```python
from build123d import *

# Parameters (mm, degrees)
F0_W        = 23
F0_H        = 25
F1_DEPTH    = 1.2
F3_DEPTH    = 25
F5_W        = 1.3906080276
F5_H        = 1.7
F5_W_2      = 1.5159434646
F6_DEPTH    = 25
F7_T1_DEPTH = 30


# Not quite as in the source:
# - a fillet or chamfer that OpenCascade refuses, or shapes differently, is made with other operations: its cross-section is extruded or revolved along the edge and cut away or added


with BuildPart() as f1:
    # F0 (on Top) → F1 (new body)
    with BuildSketch(Plane.XY):
        Rectangle(F0_W, F0_H)
    extrude(amount=F1_DEPTH)

    # F2 (on face) → F3 (join)
    with BuildSketch(Plane.XZ.offset(12.5)):
        with BuildLine():
            ThreePointArc((-8.8198933508, 1.2), (-16.4322899898, -1.1691927474), (-13.6809007153, -8.6519404997))
            Line((-13.6809007153, -8.6519404997), (-13.1818733439, -6.6722285874))
            ThreePointArc((-13.1818733439, -6.6722285874), (-14.8938387487, -2.747327312), (-11.5259407878, -0.1029107612))
            Line((-11.5259407878, -0.1029107612), (-11.5, 0))
            Line((-11.5, 0), (-11.5, 1.2))
            Line((-11.5, 1.2), (-8.8198933508, 1.2))
        make_face()
        with BuildLine():
            ThreePointArc((17, -3.4602172673), (14.1631160155, 1.3520392811), (8.578977059, 1.2))
            Line((8.578977059, 1.2), (11.5, 1.2))
            Line((11.5, 1.2), (11.5, 0.0397827327))
            ThreePointArc((11.5, 0.0397827327), (13.9748737342, -0.9853435331), (15, -3.4602172673))
            ThreePointArc((15, -3.4602172673), (14.5929628971, -5.0983810311), (13.4665254188, -6.3555199764))
            Line((13.4665254188, -6.3555199764), (14.0745145934, -8.3204512748))
            ThreePointArc((14.0745145934, -8.3204512748), (16.2122091562, -6.2966031487), (17, -3.4602172673))
        make_face()
    extrude(amount=-F3_DEPTH)

    # F5 (on face) → F6 (join)
    with BuildSketch(Plane.XZ.offset(12.5)):
        with Locations((18.6200318858, 6.0247716144)):
            Rectangle(F5_W, F5_H)
        with BuildLine():
            ThreePointArc((16.5864266455, -1.367787106), (17, -3.4602172673), (16.5864266455, -5.5526474285))
            Line((16.5864266455, -5.5526474285), (16.5864266455, -6.6252283856))
            Line((16.5864266455, -6.6252283856), (17.924727872, -6.6252283856))
            Line((17.924727872, -6.6252283856), (17.924727872, 5.1747716144))
            Line((17.924727872, 5.1747716144), (17.924727872, 6.8747716144))
            Line((17.924727872, 6.8747716144), (16.5864266455, 6.8747716144))
            Line((16.5864266455, 6.8747716144), (16.5864266455, 1.253477479))
            Line((16.5864266455, 1.253477479), (16.5864266455, -1.367787106))
        make_face()
        Polygon((32.124727872, -6.6252283856), (33.5864266455, -6.6252283856), (33.5864266455, 6.8747716144), (32.124727872, 6.8747716144), (32.124727872, 5.1747716144), align=None)
        with Locations((31.3667561397, 6.0247716144)):
            Rectangle(F5_W_2, F5_H)
        with BuildLine():
            Line((14.8461437412, -7.8252283856), (16.5864266455, -7.8252283856))
            Line((16.5864266455, -7.8252283856), (33.9574068785, -7.8252283856))
            Line((33.9574068785, -7.8252283856), (33.9574068785, -6.6252283856))
            Line((33.9574068785, -6.6252283856), (33.5864266455, -6.6252283856))
            Line((33.5864266455, -6.6252283856), (32.124727872, -6.6252283856))
            Line((32.124727872, -6.6252283856), (17.924727872, -6.6252283856))
            Line((17.924727872, -6.6252283856), (16.5864266455, -6.6252283856))
            Line((16.5864266455, -6.6252283856), (16.5864266455, -5.5526474285))
            ThreePointArc((16.5864266455, -5.5526474285), (15.8667169456, -6.8041345983), (14.8461437412, -7.8252283856))
        make_face()
        with BuildLine():
            ThreePointArc((14.333916343, 1.253477479), (15.6714164585, 0.1243726298), (16.5864266455, -1.367787106))
            Line((16.5864266455, -1.367787106), (16.5864266455, 1.253477479))
            Line((16.5864266455, 1.253477479), (14.333916343, 1.253477479))
        make_face()
    extrude(amount=-F6_DEPTH)

    # F7: fillet of radius 1 on 7 edges, made by hand

    # F7_s2 → F7_t1 (cut)
    with BuildSketch(Plane.XZ.offset(-15)):
        with BuildLine():
            ThreePointArc((33.5864266455, 5.8747716144), (33.2935334267, 6.5818783956), (32.5864266455, 6.8747716144))
            Line((32.5864266455, 6.8747716144), (33.5864266455, 6.8747716144))
            Line((33.5864266455, 6.8747716144), (33.5864266455, 5.8747716144))
        make_face()
        with BuildLine():
            ThreePointArc((17.5864266455, 6.8747716144), (16.8793198643, 6.5818783956), (16.5864266455, 5.8747716144))
            Line((16.5864266455, 5.8747716144), (16.5864266455, 6.8747716144))
            Line((16.5864266455, 6.8747716144), (17.5864266455, 6.8747716144))
        make_face()
        with BuildLine():
            ThreePointArc((18.3153358996, 5.1747716144), (19.0224426808, 5.4676648332), (19.3153358996, 6.1747716144))
            Line((19.3153358996, 6.1747716144), (19.3153358996, 5.1747716144))
            Line((19.3153358996, 5.1747716144), (18.3153358996, 5.1747716144))
        make_face()
        with BuildLine():
            ThreePointArc((30.6087844074, 6.1747716144), (30.9016776262, 5.4676648332), (31.6087844074, 5.1747716144))
            Line((31.6087844074, 5.1747716144), (30.6087844074, 5.1747716144))
            Line((30.6087844074, 5.1747716144), (30.6087844074, 6.1747716144))
        make_face()
        with BuildLine():
            ThreePointArc((31.6087844074, 6.8747716144), (30.9016776262, 6.5818783956), (30.6087844074, 5.8747716144))
            Line((30.6087844074, 5.8747716144), (30.6087844074, 6.8747716144))
            Line((30.6087844074, 6.8747716144), (31.6087844074, 6.8747716144))
        make_face()
        with BuildLine():
            ThreePointArc((18.3153358996, 6.8747716144), (19.0224426808, 6.5818783956), (19.3153358996, 5.8747716144))
            Line((19.3153358996, 5.8747716144), (19.3153358996, 6.8747716144))
            Line((19.3153358996, 6.8747716144), (18.3153358996, 6.8747716144))
        make_face()
        with BuildLine():
            ThreePointArc((32.9574068785, -7.8252283856), (33.6645136597, -7.5323351668), (33.9574068785, -6.8252283856))
            Line((33.9574068785, -6.8252283856), (33.9574068785, -7.8252283856))
            Line((33.9574068785, -7.8252283856), (32.9574068785, -7.8252283856))
        make_face()
    extrude(amount=F7_T1_DEPTH, mode=Mode.SUBTRACT)


solid = f1.part
```
Design review of the part built by this model. Coordinates are the model's own, in mm. A direction names the side the tool comes from. Give positions to 0.01 mm unless a question says otherwise; leave off trailing zeros. Loops run counter-clockwise (first coordinate to the right, second up) from the corner with the lowest first, then second, coordinate; pieces in that order, holes last. Notation, with made-up numbers: (85, 31) -> (90, 31) arc R18 cw to (90, 65) -> close; hole circle Ø5 at (82.5, 21). An arc over 180 degrees is marked (long way). One line per item, written item: value.
Q1. For L1, parallel to X at y = -8, z = -3.5; L2, parallel to Z at x = 32, y = -4; L3, parallel to X at y = 3.25, z = -3, list the stretches that pass through material, from the lowest coordinate up.
Numbers:
L1: x = -17 to -15, 15 to 17.92, 32.12 to 33.59
L2: z = -7.83 to -6.63, 5.17 to 6.87
L3: x = -16.97 to -14.95, 14.97 to 17.92, 32.12 to 33.59
Q2. We need section A-A on z = 4. Give the boundary of the cut face in (x, y), and give its area (3 significant figures).
Numbers:
outline: (16.59, -12.5) -> (17.92, -12.5) -> (17.92, 12.5) -> (16.59, 12.5) -> close; (32.12, -12.5) -> (33.59, -12.5) -> (33.59, 12.5) -> (32.12, 12.5) -> close
area: 70.0 mm^2
Q3. Machinability: for faces 5 (the flat face through (15, 0, 1.253)), 6 (the cylindrical face through (-14.91, -0.18, -2.81)), 7 (the flat face through (13.766, -0.175, -7.324)), which of the approach directions +Z, -Z, +X, -X, +Y, -Y give a long, thin tool a straight path to every point of the face, cutting with its end or side? Answer none if there is none.
Numbers:
face 5: +Z, +Y, -Y
face 6: +Y, -Y
face 7: -Z, +Y, -Y
Q4. We need section D-D on x = -3. Give the boundary of the cut face in (y, z), and give its area (3 significant figures).
Numbers:
outline: (-12.5, 0) -> (12.5, 0) -> (12.5, 1.2) -> (-12.5, 1.2) -> close
area: 30.0 mm^2
Q5. We need section C-C on z = -4. Give the boundary of the cut face in (x, y).
Numbers:
outline: (-16.99, -12.5) -> (-14.98, -12.5) -> (-14.98, 12.5) -> (-16.99, 12.5) -> close; (14.96, -12.5) -> (17.92, -12.5) -> (17.92, 12.5) -> (14.96, 12.5) -> close; (32.12, -12.5) -> (33.59, -12.5) -> (33.59, 12.5) -> (32.12, 12.5) -> close
Q6. For pin 1 Ø5 at (y, z) = (6.5, 3) entering from +X; pin 2 Ø8 at (x, z) = (12.5, 2) entering from +Y; pin 3 Ø5 at (x, y) = (0, 10) entering from +Z; pin 4 Ø9 at (x, y) = (19.5, -2.5) entering from -Z, all flat-tipped, find the tip position at first contact; note any pin that passes through.
Numbers:
pin 1: stops at x = 33.59
pin 2: stops at y = 12.5
pin 3: stops at z = 1.2
pin 4: stops at z = -7.83
Q7. Draft analysis for pull direction X (two halves, no side actions). For faces 1 (the cylindrical face through (18.96, 0.18, 6.64)), 2 (the cylindrical face through (18.96, 0.18, 5.41)), 3 (the cylindrical face through (33.301, 0.175, 6.574)), 4 (the cylindrical face through (16.9, 0.2, 6.6)), state which applies: pulls with the +X half, pulls with the -X half, needs draft (parallel to the pull), parting line crosses it, or undercut.
Numbers:
face 1: undercut
face 2: undercut
face 3: pulls with the +X half
face 4: pulls with the -X half
